```python
from build123d import *

# Parameters (mm, degrees)
SKETCH1_W           = 744
SKETCH1_H           = 590
BOSS_EXTRUDE1_DEPTH = 695
BOSS_EXTRUDE1_TAPER = 15
SKETCH6_W           = 734
SKETCH6_H           = 580
CUT_EXTRUDE3_DEPTH  = 784
CUT_EXTRUDE3_DRAFT  = -15
SKETCH7_W           = 371.55062252
SKETCH7_H           = 217.55062252
BOSS_EXTRUDE2_DEPTH = 251
SKETCH8_R           = 10
CUT_EXTRUDE4_DEPTH  = 100


with BuildPart() as part:
    # Sketch1 → Boss-Extrude1 (new body)
    with BuildSketch(Plane(origin=(0, 0, 0), x_dir=(1, 0, 0), z_dir=(0, 1, 0))):
        with Locations((372, 295)):
            Rectangle(SKETCH1_W, SKETCH1_H)
    extrude(amount=BOSS_EXTRUDE1_DEPTH, taper=BOSS_EXTRUDE1_TAPER)


with BuildPart() as cut_extrude3_tool:
    # Sketch6 → Cut-Extrude3 (with draft: the straight prism first)
    with BuildSketch(Plane.XZ):
        with Locations((372, -295)):
            Rectangle(SKETCH6_W, SKETCH6_H)
    extrude(amount=-CUT_EXTRUDE3_DEPTH)
    # Cut-Extrude3: the draft: its side faces are tilted about the plane it starts from
    cut_extrude3_sides = [cut_extrude3_tool.faces().sort_by_distance(p)[0] for p in [
        (372, 392, -585),
        (739, 392, -295),
        (372, 392, -5),
        (5, 392, -295),
    ]]
    draft(cut_extrude3_sides, Plane.XZ, CUT_EXTRUDE3_DRAFT)


with BuildPart() as part_1:
    add(part.part)

    # Cut-Extrude3: cut by cut_extrude3_tool
    add(cut_extrude3_tool.part, mode=Mode.SUBTRACT)

    # Sketch7 → Boss-Extrude2 (add)
    with BuildSketch(Plane(origin=(0, 695, 0), x_dir=(1, 0, 0), z_dir=(0, 1, 0))):
        with Locations((372, 295)):
            Rectangle(SKETCH7_W, SKETCH7_H)
    extrude(amount=BOSS_EXTRUDE2_DEPTH)

    # Sketch8 → Cut-Extrude4 (cut)
    with BuildSketch(Plane.XY.offset(-186.22468874)):
        with Locations((372, 879)):
            Circle(SKETCH8_R)
    extrude(amount=-CUT_EXTRUDE4_DEPTH, mode=Mode.SUBTRACT)


solid = part_1.part
```
CAD build for the part. Positions are in the model's coordinates, mm. A direction names the side the tool comes from. Round coordinates to 2 decimals unless told otherwise and drop trailing zeros.
Item 1: Mould opens along Z. For faces 5 (the face through (369, 819, -403.775)), 6 (the face through (366.862, 265.413, -76.117)), 7 (the face through (369, 946, -297)) say: pulls with the +Z half, pulls with the -Z half, needs draft (parallel to the pull), parting line crosses it, or undercut.
Item 2: Pin check, flat tips, straight feed: pin 1 (5 mm diameter, centred on x = 444, y = 598.5, fed in from +Z); pin 2 (22 mm diameter, centred on x = 376.5, y = 875, fed in from +Z); pin 3 (3 mm diameter, centred on x = 321.5, y = 282.5, fed in from +Z). Stop position of each tip, or through.
Item 3: Probe line 1 along Y through (x, z) = (372, -223); line 2 along X through (y, z) = (879, -230); line 3 along Z through (x, y) = (328.5, 634). List the from-to ranges inside material, lowest first.
Item 4: Tool access for faces 1 (the face through (667.883, 265.413, -299.06)), 2 (the face through (369, 819, -186.225)), 3 (the face through (557.775, 819, -293)), 4 (the face through (186.225, 819, -293)): list every direction of +Z, -Z, +X, -X, +Y, -Y with a clear straight run to the whole face (end or side of a thin tool).
Reported:
1. face 5: pulls with the -Z half
1. face 6: undercut
1. face 7: needs draft
2. pin 1: stops at z = -159.7
2. pin 2: stops at z = -186.22
2. pin 3: stops at z = -75.29
3. line 1: y = 695 to 869, 889 to 946
3. line 2: x = 186.22 to 362, 382 to 557.78
3. line 3: z = -420.12 to -415.12, -174.88 to -169.88
4. face 1: -Y
4. face 2: +Z, +X, -X, +Y
4. face 3: +Z, -Z, +X, +Y
4. face 4: +Z, -Z, -X, +Y
